Source: CAD feature listing. Evaluate the final solid. Frame: model axes, mm. A direction names the side the tool comes from. Give positions to 0.01 mm unless a question says otherwise; leave off trailing zeros. Loops run counter-clockwise (first coordinate to the right, second up) from the corner with the lowest first, then second, coordinate; pieces in that order, holes last.
from build123d import *

# Parameters (mm, degrees)
PAD002_DEPTH = 36.02
PAD003_DEPTH = 36.02
PAD004_DEPTH = 36.02
PAD001_DEPTH = 36.02
SKETCH005_R  = 2.5
PAD005_DEPTH = 3.05
SKETCH006_R  = 6.606667
PAD006_DEPTH = 2.33
PAD_DEPTH    = 19.82
FILLET_R     = 1


with BuildPart() as body002:
    # Sketch002 → Pad002 (new body)
    with BuildSketch(Plane.XZ):
        with BuildLine():
            ThreePointArc((-32.39, 17.185), (-34.58, 14.995), (-32.39, 12.805))
            Line((-32.39, 12.805), (-23.63, 12.805))
            ThreePointArc((-23.63, 12.805), (-21.44, 14.995), (-23.63, 17.185))
            Line((-32.39, 17.185), (-23.63, 17.185))
        make_face()
    extrude(amount=-PAD002_DEPTH)


with BuildPart() as body003:
    # Sketch003 → Pad003 (new body)
    with BuildSketch(Plane.XZ):
        with BuildLine():
            ThreePointArc((23.63, 7.015), (21.44, 4.825), (23.63, 2.635))
            Line((23.63, 2.635), (32.39, 2.635))
            ThreePointArc((32.39, 2.635), (34.58, 4.825), (32.39, 7.015))
            Line((23.63, 7.015), (32.39, 7.015))
        make_face()
    extrude(amount=-PAD003_DEPTH)


with BuildPart() as body004:
    # Sketch004 → Pad004 (new body)
    with BuildSketch(Plane.XZ):
        with BuildLine():
            ThreePointArc((23.63, 17.185), (21.44, 14.995), (23.63, 12.805))
            Line((23.63, 12.805), (32.39, 12.805))
            ThreePointArc((32.39, 12.805), (34.58, 14.995), (32.39, 17.185))
            Line((23.63, 17.185), (32.39, 17.185))
        make_face()
    extrude(amount=-PAD004_DEPTH)


with BuildPart() as fusion:
    # Sketch001 → Pad001 (new body)
    with BuildSketch(Plane.XZ):
        with BuildLine():
            ThreePointArc((-32.39, 7.015), (-34.58, 4.825), (-32.39, 2.635))
            Line((-32.39, 2.635), (-23.63, 2.635))
            ThreePointArc((-23.63, 2.635), (-21.44, 4.825), (-23.63, 7.015))
            Line((-32.39, 7.015), (-23.63, 7.015))
        make_face()
    extrude(amount=-PAD001_DEPTH)

    # Fusion: union Body002, Body003, Body004
    add(body002.part)
    add(body003.part)
    add(body004.part)


with BuildPart() as body005:
    # Sketch005 → Pad005 (new body)
    with BuildSketch(Plane.XZ):
        with Locations((10.28, 9.91)):
            Circle(SKETCH005_R)
    extrude(amount=-PAD005_DEPTH)


with BuildPart() as body005_1:
    # Body005 placement: moved
    add(body005.part.moved(Location((0, 38.35, 0))))


with BuildPart() as body006:
    # Sketch006 → Pad006 (new body)
    with BuildSketch(Plane.XZ):
        with Locations((10.28, 9.91)):
            Circle(SKETCH006_R)
    extrude(amount=-PAD006_DEPTH)


with BuildPart() as body006_1:
    # Body006 placement: moved
    add(body006.part.moved(Location((0, 36.02, 0))))


with BuildPart() as cut:
    # Sketch → Pad (new body)
    with BuildSketch(Plane.XY):
        Polygon((-19.94, 0), (-19.94, 26.67), (-26.42, 26.67), (-26.42, 28.67), (-19.94, 28.67), (-19.94, 36.02), (19.94, 36.02), (19.94, 28.67), (26.42, 28.67), (26.42, 26.67), (19.94, 26.67), (19.94, 0), align=None)
    extrude(amount=PAD_DEPTH)

    # Fillet
    fillet_edges = [cut.edges().sort_by_distance(p)[0] for p in [
        (0, 36.02, 19.82),
        (0, 36.02, 0),
        (-19.94, 36.02, 9.91),
        (-19.94, 32.345, 0),
        (-19.94, 32.345, 19.82),
        (-19.94, 13.335, 0),
        (-19.94, 13.335, 19.82),
        (-19.94, 0, 9.91),
        (0, 0, 0),
        (19.94, 13.335, 0),
        (19.94, 32.345, 0),
        (19.94, 36.02, 9.91),
        (19.94, 32.345, 19.82),
        (19.94, 13.335, 19.82),
        (19.94, 0, 9.91),
        (0, 0, 19.82),
    ]]
    fillet(fillet_edges, radius=FILLET_R)

    # Fusion001: union Body005, Body006
    add(body005_1.part)
    add(body006_1.part)

    # Cut: cut Fusion
    add(fusion.part, mode=Mode.SUBTRACT)


solid = cut.part
1) Cut plane C-C (z = 1.75). Return loops of the section in (x, y), and give its area (3 significant figures).
Checks:
outline: (-26.42, 26.67) - (-19.94, 26.67) - (-19.94, 1) arc R1 ccw to (-18.94, 0) - (18.94, 0) arc R1 ccw to (19.94, 1) - (19.94, 26.67) - (26.42, 26.67) - (26.42, 28.67) - (19.94, 28.67) - (19.94, 35.02) arc R1 ccw to (18.94, 36.02) - (-18.94, 36.02) arc R1 ccw to (-19.94, 35.02) - (-19.94, 28.67) - (-26.42, 28.67) - close
area: 1,460 mm2
2) Contact query for flat-ended pins moving along their axis: P1, Ø10, axis at x = -4.5, z = 9.5, coming from the +Y side; P2, Ø3.5, axis at x = -22, z = 9.5, coming from the -Y side; P3, Ø7, axis at y = 32.5, z = 14, coming from the -X side. Output: stop coordinate, or through.
Checks:
P1: stops at y = 36.02
P2: stops at y = 26.67
P3: stops at x = -19.94
3) Cut plane D-D (x = 23). Return loops of the section in (y, z).
Checks:
outline: (26.67, 0) - (28.67, 0) - (28.67, 2.73) - (26.67, 2.73) - close; (26.67, 6.92) - (28.67, 6.92) - (28.67, 12.9) - (26.67, 12.9) - close; (26.67, 17.09) - (28.67, 17.09) - (28.67, 19.82) - (26.67, 19.82) - close
4) Reachability of faces 5 (the flat face through (-25, 28, 12.805)), 6 (the flat face through (13, 38.35, 10)), 7 (the flat face through (-19.94, 32, 10)), 8 (the flat face through (25, 28, 17.185)), 9 (the flat face through (26.42, 28, 1)) from +Z, -Z, +X, -X, +Y, -Y: full face, straight path, thin tool, end or side. Return the list, or none.
Checks:
face 5: -X, +Y, -Y
face 6: +Y
face 7: +Z, -Z, -X, +Y
face 8: +X, +Y, -Y
face 9: +Z, -Z, +X, +Y, -Y
5) Pull-direction query (Z, two-part tool) for faces 1 (the cylindrical face through (-21.44, 27.66, 14.95)), 2 (the cylindrical face through (9.42, 37.17, 16.46)), 3 (the flat face through (0, 18, 19.82)), 4 (the flat face through (25, 28, 2.635)); classes: released by +Z, released by -Z, zero draft, split by the parting line, or undercut.
Checks:
face 1: undercut
face 2: split by the parting line
face 3: released by +Z
face 4: undercut
6) Ray query, probe 1 along X at (y, z) = (18.5, 15.75); probe 2 along Y at (x, z) = (16, 6.25); probe 3 along Y at (x, z) = (13.5, 10.5). Return the intervals inside material, ascending.
Checks:
probe 1: x = -19.94 to 19.94
probe 2: y = 0 to 36.02
probe 3: y = 0 to 38.35
7) Cut plane A-A (x = -2). Return loops of the section in (y, z).
Checks:
outline: (0, 1) arc R1 ccw to (1, 0) - (35.02, 0) arc R1 ccw to (36.02, 1) - (36.02, 18.82) arc R1 ccw to (35.02, 19.82) - (1, 19.82) arc R1 ccw to (0, 18.82) - close
8) Cut plane B-B (y = 18.5). Return loops of the section in (x, z).
Checks:
outline: (-19.94, 1) arc R1 ccw to (-18.94, 0) - (18.94, 0) arc R1 ccw to (19.94, 1) - (19.94, 18.82) arc R1 ccw to (18.94, 19.82) - (-18.94, 19.82) arc R1 ccw to (-19.94, 18.82) - close
